```python
from build123d import *

# Parameters (mm, degrees)
F1_DEPTH = 12.7
F2_DEPTH = 7.62
F3_R     = 5.08
F4_R     = 5.08
F5_R     = 1.27
F6_R     = 1.27


with BuildPart() as f1:
    # F0 (on Top) → F1 (new body)
    with BuildSketch(Plane.XY):
        with BuildLine():
            ThreePointArc((274.3839541464, 271.162187256), (356.8357568685, 146.5732878479), (385.7661028272, 0))
            Line((385.7661028272, 0), (394.4020265055, 0))
            ThreePointArc((394.4020265055, 0), (364.7896986096, 149.9381015618), (280.3993957424, 277.3610235395))
            Line((280.3993957424, 277.3610235395), (274.3839541464, 271.162187256))
        make_face()
        with BuildLine():
            ThreePointArc((280.3993957424, 277.3610235395), (364.7896986096, 149.9381015618), (394.4020265055, 0))
            Line((394.4020265055, 0), (453.5602591088, 0))
            ThreePointArc((453.5602591088, 0), (419.2757542113, 172.9877179841), (321.6053535703, 319.8232405529))
            Line((321.6053535703, 319.8232405529), (280.3993957424, 277.3610235395))
        make_face()
        with BuildLine():
            ThreePointArc((321.6053535703, 319.8232405529), (419.2757542113, 172.9877179841), (453.5602591088, 0))
            Line((453.5602591088, 0), (462.3607499635, 0))
            ThreePointArc((462.3607499635, 0), (427.3811495561, 176.4165981731), (327.7350659564, 326.1398314365))
            Line((327.7350659564, 326.1398314365), (321.6053535703, 319.8232405529))
        make_face()
    extrude(amount=F1_DEPTH)

    # F0 (on Top) → F2 (cut)
    with BuildSketch(Plane.XY):
        with BuildLine():
            ThreePointArc((280.3993957424, 277.3610235395), (364.7896986096, 149.9381015618), (394.4020265055, 0))
            Line((394.4020265055, 0), (453.5602591088, 0))
            ThreePointArc((453.5602591088, 0), (419.2757542113, 172.9877179841), (321.6053535703, 319.8232405529))
            Line((321.6053535703, 319.8232405529), (280.3993957424, 277.3610235395))
        make_face()
        with BuildLine():
            Line((453.5602591088, 0), (394.4020265055, 0))
            ThreePointArc((394.4020265055, 0), (-364.7896986096, -149.9381015618), (280.3993957424, 277.3610235395))
            Line((280.3993957424, 277.3610235395), (321.6053535703, 319.8232405529))
            ThreePointArc((321.6053535703, 319.8232405529), (-419.2757542113, -172.9877179841), (453.5602591088, 0))
        make_face()
    extrude(amount=F2_DEPTH, mode=Mode.SUBTRACT)

    # F3
    f3_edges = [f1.edges().sort_by_distance(p)[0] for p in [
        (427.38115, 176.416598, 0),
    ]]
    fillet(f3_edges, radius=F3_R)

    # F4
    f4_edges = [f1.edges().sort_by_distance(p)[0] for p in [
        (356.835757, 146.573288, 0),
    ]]
    fillet(f4_edges, radius=F4_R)

    # F5
    f5_edges = [f1.edges().sort_by_distance(p)[0] for p in [
        (427.38115, 176.416598, 12.7),
    ]]
    fillet(f5_edges, radius=F5_R)

    # F6
    f6_edges = [f1.edges().sort_by_distance(p)[0] for p in [
        (356.835757, 146.573288, 12.7),
    ]]
    fillet(f6_edges, radius=F6_R)


solid = f1.part
```
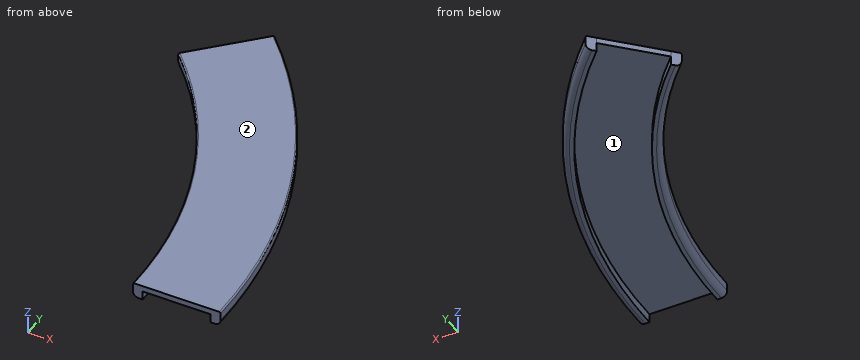
The model under review builds one solid part; all positions refer to its coordinate system, in mm. Face numbers are marked on the shaded views. Give positions to 0.01 mm unless a question says otherwise; leave off trailing zeros. Write each loop counter-clockwise with the first axis right and the second up, starting at its lowest first coordinate (ties: lowest second). Pieces come first, ordered by that corner, then holes. Notation, with made-up numbers: (30, 66) -> (55, 66) arc R17 cw to (55, 87) -> close; hole circle Ø1 at (14.5, -15). An arc over 180 degrees is marked (long way). Answer in a Markdown table with one row per item.
1) Add section A-A on z = 2.25. State the section outline as (x, y) points, plus the area to 3 significant figures.
Worked answers:
| item | result |
|---|---|
| outline | (274.98, 271.78) arc R386.63 cw to (386.63, 0) -> (394.4, 0) arc R394.4 ccw to (280.4, 277.36) -> close; (321.61, 319.82) arc R453.56 cw to (453.56, 0) -> (461.5, 0) arc R461.5 ccw to (327.14, 325.52) -> close |
| area | 5,210 mm² |
2) Mouldability with a two-part tool opening along Y and no side actions: class the marked faces 1 and 2 as +Y half, -Y half, draft (parallel to the pull), parting line (faces both ways), or undercut.
Worked answers:
| item | result |
|---|---|
| face 1 | undercut |
| face 2 | draft |
3) For L1, parallel to Z at x = 407, y = 142; L2, parallel to X at y = 44.5, z = 3.25; L3, parallel to X at y = 179, z = 4, list the stretches that pass through material, from the lowest coordinate up. Write a range as [from, to].
Worked answers:
| item | result |
|---|---|
| L1 | [7.62, 12.7] |
| L2 | [383.53, 391.88], [451.37, 459.87] |
| L3 | [341.85, 351.44], [416.74, 426.18] |
4) Clearance check with flat-ended pins moving along their axes: P1, Ø1.5, axis at y = 289, z = 5.5, coming from the -X side; P2, Ø3, axis at x = 301, z = 1.5, coming from the -Y side; P3, Ø3, axis at y = 245.5, z = 7.5, coming from the +X side. State where each tip first meets the part, or that it passes through.
Worked answers:
| item | result |
|---|---|
| P1 | x = 348.94 |
| P2 | y = 241 |
| P3 | x = 392.74 |
